```python
from build123d import *

# Parameters (mm, degrees)
SKETCH_1_W          = 75
SKETCH_1_H          = 75
EXTRUDE_1_DEPTH     = 15
SKETCH_2_R          = 2
CUT_EXTRUDE_1_DEPTH = 15
SKETCH_3_R          = 2
CUT_EXTRUDE_2_DEPTH = 56.113519213
FILLET_1_R          = 10
CUT_EXTRUDE_4_DEPTH = 15
CUT_EXTRUDE_5_DEPTH = 56.113519213
FILLET_3_R          = 5
FILLET_4_R          = 3
SKETCH_6_R          = 2
CUT_EXTRUDE_6_DEPTH = 15
SKETCH_8_W          = 15
SKETCH_8_H          = 15
EXTRUDE_2_DEPTH     = 15
FILLET_5_R          = 3
SKETCH_9_R          = 2
CUT_EXTRUDE_8_DEPTH = 93.769876576


with BuildPart() as part:
    # 草图1 → 凸台-拉伸1 (new body)
    with BuildSketch(Plane.XY):
        Rectangle(SKETCH_1_W, SKETCH_1_H)
    extrude(amount=EXTRUDE_1_DEPTH)

    # 草图2 → 切除-拉伸1 (cut)
    with BuildSketch(Plane.XY.offset(15)):
        with Locations((-20, 31.5)):
            Circle(SKETCH_2_R)
        with Locations((20, 31.5)):
            Circle(SKETCH_2_R)
        with Locations((20, -31.5)):
            Circle(SKETCH_2_R)
        with Locations((-20, -31.5)):
            Circle(SKETCH_2_R)
    extrude(amount=-CUT_EXTRUDE_1_DEPTH, mode=Mode.SUBTRACT)

    # 草图3 → 切除-拉伸2 (cut, through all)
    with BuildSketch(Plane.XY.offset(15)):
        with Locations((-31.5, 20)):
            Circle(SKETCH_3_R)
        with Locations((-31.5, -20)):
            Circle(SKETCH_3_R)
        with Locations((31.5, -20)):
            Circle(SKETCH_3_R)
        with Locations((31.5, 20)):
            Circle(SKETCH_3_R)
    extrude(amount=-CUT_EXTRUDE_2_DEPTH, mode=Mode.SUBTRACT)

    # 圆角1
    fillet_1_edges = [part.edges().sort_by_distance(p)[0] for p in [
        (37.5, -37.5, 7.5),
        (-37.5, -37.5, 7.5),
    ]]
    fillet(fillet_1_edges, radius=FILLET_1_R)

    # 草图4 → 切除-拉伸4 (cut)
    with BuildSketch(Plane.XY.offset(15)):
        Polygon((-5.656854249, -5.656854249), (-22.5, 11.186291501), (-22.5, -22.5), align=None)
        Polygon((0, -11.313708499), (-11.186291501, -22.5), (11.186291501, -22.5), align=None)
        Polygon((22.5, -22.5), (22.5, 11.186291501), (5.656854249, -5.656854249), align=None)
    extrude(amount=-CUT_EXTRUDE_4_DEPTH, mode=Mode.SUBTRACT)

    # 草图5 → 切除-拉伸5 (cut, through all)
    with BuildSketch(Plane.XY.offset(15)):
        Polygon((22.5, 22.5), (-22.5, 22.5), (-22.5, 14.5), (0, 0.5), (22.5, 14.5), align=None)
    extrude(amount=-CUT_EXTRUDE_5_DEPTH, mode=Mode.SUBTRACT)

    # 圆角3
    fillet_3_edges = [part.edges().sort_by_distance(p)[0] for p in [
        (22.5, 11.186291501, 7.5),
        (-22.5, 11.186291501, 7.5),
    ]]
    fillet(fillet_3_edges, radius=FILLET_3_R)

    # 圆角4
    fillet_4_edges = [part.edges().sort_by_distance(p)[0] for p in [
        (22.5, 14.5, 7.5),
        (0, 0.5, 7.5),
        (-22.5, 14.5, 7.5),
        (-22.5, 22.5, 7.5),
        (22.5, 22.5, 7.5),
        (-11.186291501, -22.5, 7.5),
        (0, -11.313708499, 7.5),
        (11.186291501, -22.5, 7.5),
        (5.656854249, -5.656854249, 7.5),
        (22.5, -22.5, 7.5),
        (-5.656854249, -5.656854249, 7.5),
        (-22.5, -22.5, 7.5),
    ]]
    fillet(fillet_4_edges, radius=FILLET_4_R)

    # 草图6 → 切除-拉伸6 (cut)
    with BuildSketch(Plane(origin=(0, 37.5, 0), x_dir=(1, 0, 0), z_dir=(0, 1, 0))):
        with Locations(Location((-14, -7.5, 0), (0, 0, 270))):
            Circle(SKETCH_6_R)
        with Locations(Location((14, -7.5, 0), (0, 0, 90))):
            Circle(SKETCH_6_R)
    extrude(amount=-CUT_EXTRUDE_6_DEPTH, mode=Mode.SUBTRACT)

    # 草图8 → 凸台-拉伸2 (add)
    with BuildSketch(Plane.XY.offset(15)):
        with Locations((-45, 30)):
            Rectangle(SKETCH_8_W, SKETCH_8_H)
        with Locations((45, 30)):
            Rectangle(SKETCH_8_W, SKETCH_8_H)
    extrude(amount=-EXTRUDE_2_DEPTH)

    # 圆角5
    fillet_5_edges = [part.edges().sort_by_distance(p)[0] for p in [
        (-37.5, 22.5, 7.5),
        (37.5, 22.5, 7.5),
    ]]
    fillet(fillet_5_edges, radius=FILLET_5_R)

    # 草图9 → 切除-拉伸8 (cut, through all)
    with BuildSketch(Plane(origin=(0, 37.5, 0), x_dir=(1, 0, 0), z_dir=(0, 1, 0))):
        with Locations(Location((-47.5, -7.5, 0), (0, 0, 270))):
            Circle(SKETCH_9_R)
        with Locations((47.5, -7.5)):
            Circle(SKETCH_9_R)
    extrude(amount=-CUT_EXTRUDE_8_DEPTH, mode=Mode.SUBTRACT)


solid = part.part
```
Source: CAD feature listing. Evaluate the final solid. Frame: model axes, mm. A direction names the side the tool comes from. Coordinates: 2 decimals unless noted, no trailing zeros. Order: outer loops, then holes, each group sorted by start corner. A loop starts at its lowest first (then second) coordinate and runs counter-clockwise, first axis right, second up. Notation, with made-up numbers: M 11.5,23.5 L 37.5,23.5 A20 ccw 37.5,52.5 Z; hole C -16,81.25 d8. An arc over 180 degrees is marked long. Write each question's results on one line, items separated by ' | '. Start each with the question number.
1) Section query B-B (x = 47.5). Return the cut outline in (y, z).
2) Section query C-C (z = 7.5). Give the number of separate pieces and of enclosed holes in the cut face, plus the area to 3 significant figures.
3) Contact query for flat-ended pins moving along their axis: pin 1 Ø1.7 at (y, z) = (18.5, 11) entering from +X; pin 2 Ø3 at (x, z) = (14, 7.5) entering from +Y; pin 3 Ø1.5 at (x, z) = (36, 3.5) entering from -Y. Output: stop coordinate, or through.
4) Access query for faces 1 (the face through (37.5, -4, 7)), 2 (the face through (-6.9, -5.6, 7.4)), 3 (the face through (-12.648, 30.105, 6.026)). Directions: +Z, -Z, +X, -X, +Y, -Y. A direction counts if a zero-diameter tool reaches every point of the face in a straight line with its end or side. Return the directions, or none.
5) Section query A-A (y = 31.5). Return the cut outline in (x, z).
6) Draft query along Z for faces 4 (the face through (-1, 1, 0)), 5 (the face through (-49.452, 30.105, 7.066)), 6 (the face through (11.2, 7.47, 7.6)). Return one class per face: released by +Z, released by -Z, zero draft, split by the parting line, or undercut.
7) Section query D-D (y = -6). Return the cut outline in (x, z), plus the area to 3 significant figures.
8) Line query: line 1 (X direction, y = 27, z = 7.5); line 2 (Y direction, x = -31.5, z = 6); line 3 (Y direction, x = 15.5, z = 10). Output: solid intervals per line, ascending. Write a range as from..to.
Answers:
1) outline: M 22.5,0 L 37.5,0 L 37.5,5.5 L 22.5,5.5 Z; M 22.5,9.5 L 37.5,9.5 L 37.5,15 L 22.5,15 Z
2) separate pieces: 4 | enclosed holes: 11 | area: 4,450 mm^2
3) pin 1: stops at x = 37.5 | pin 2: stops at y = 10.14 | pin 3: stops at y = -33.82
4) face 1: +Z, -Z, +X, -Y | face 2: +Z, -Z | face 3: +Y
5) outline: M -52.5,0 L -22,0 L -22,15 L -52.5,15 Z; M -18,0 L 18,0 L 18,15 L -18,15 Z; M 22,0 L 52.5,0 L 52.5,15 L 22,15 Z; hole C -47.5,7.5 d4; hole C -14,7.5 d4; hole C 14,7.5 d4; hole C 47.5,7.5 d4
6) face 4: released by -Z | face 5: undercut | face 6: zero draft
7) outline: M -37.5,0 L -22.5,0 L -22.5,15 L -37.5,15 Z; M -6.92,0 L 6.92,0 L 6.92,15 L -6.92,15 Z; M 22.5,0 L 37.5,0 L 37.5,15 L 22.5,15 Z | area: 658 mm^2
8) line 1: x = -52.5..-49.5, -45.5..-16, -12..12, 16..45.5, 49.5..52.5 | line 2: y = -36.67..-22, -18..18, 22..37.5 | line 3: y = -37.5..-15.5, 3.7..10.14, 22.5..37.5
